Job drawing, mm, ordinate dimensions from the low corner. One solid piece. A direction names the side the tool comes from. Give positions to 0.01 mm unless a question says otherwise; leave off trailing zeros. Order: outer loops, then holes, each group sorted by start corner. A loop starts at its lowest first (then second) coordinate and runs counter-clockwise, first axis right, second up. Notation, with made-up numbers: (48, 14.5) - (96, 14.5) arc R35 ccw to (96, 49.5) - close; hole circle Ø8 at (65.5, 19). An arc over 180 degrees is marked (long way). Use one line per item in the form item = value. Start each with the question number.
1. Band-saw the part on D-D, the plane y = 16. List the corners of the cut face in (x, z).
2. Band-saw the part on C-C, the plane z = 23. List the corners of the cut face in (x, y).
3. Band-saw the part on A-A, the plane y = 7.5. List the corners of the cut face in (x, z).
4. Tool access for the marked faces 1, 2 and 3: list every direction of +Z, -Z, +X, -X, +Y, -Y with a clear straight run to the whole face (end or side of a thin tool).
5. Band-saw the part on B-B, the plane z = 41. List the corners of the cut face in (x, y), plus the area to 3 significant figures.
6. Pin check, flat tips, straight feed: P1, Ø8, axis at x = 33, z = 39, coming from the +Y side; P2, Ø12, axis at x = 28.5, z = 9, coming from the +Y side; P3, Ø1.5, axis at x = 26.5, z = 15.5, coming from the +Y side. Stop position of each tip, or through.
7. Drill centre lines: line 1 (Z direction, x = 37.5, y = 28); line 2 (Y direction, x = 29, z = 28.5); line 3 (X direction, y = 6.5, z = 41.5). Where is each one in solid material? Low to high.
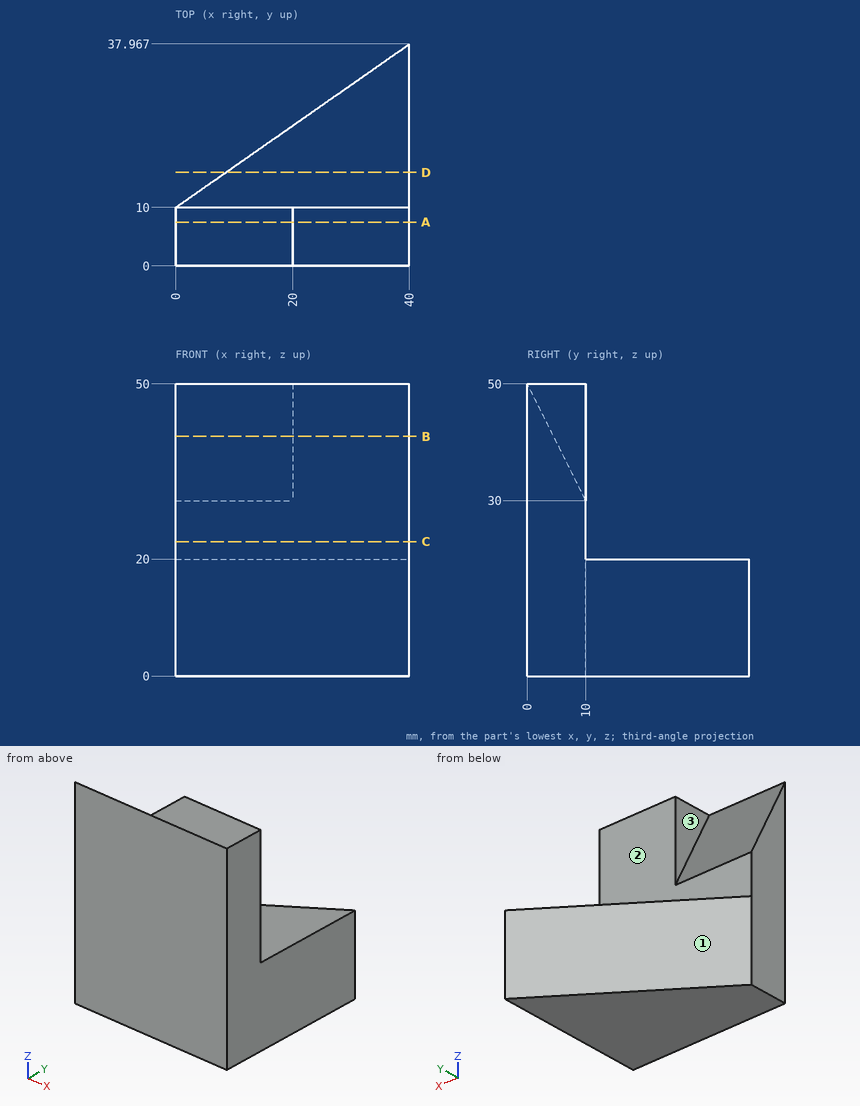
From the geometry:
q1.outline = (8.58, 0) - (40, 0) - (40, 20) - (8.58, 20) - close
q2.outline = (0, 0) - (40, 0) - (40, 10) - (0, 10) - close
q3.outline = (0, 0) - (40, 0) - (40, 50) - (20, 50) - (20, 35) - (0, 35) - close
q4.face_1 = +Z, -Z, -X, +Y
q4.face_2 = +Z, +X, -X, +Y
q4.face_3 = +Z, -X, +Y
q5.outline = (0, 0) - (40, 0) - (40, 10) - (20, 10) - (20, 4.5) - (0, 4.5) - close
q5.area = 290 mm²
q6.P1 = 10
q6.P2 = 34.12
q6.P3 = 29.05
q7.line_1 = 0 to 20
q7.line_2 = 0 to 10
q7.line_3 = 20 to 40
